Autodesk Inventor part; units mm, degrees
ref_plane "YZ Plane" through (0, 0, 0) normal (1, 0, 0) x (0, 1, 0)
ref_plane "XZ Plane" through (0, 0, 0) normal (0, 1, 0) x (-1, 0, 0)
ref_plane "XY Plane" through (0, 0, 0) normal (0, 0, 1) x (1, 0, 0)
sketch "Sketch1" plane through (0, 0, 0) normal (0, 0, 1) x (1, 0, 0)
  line L0 (-17.5, 16) -> (17.5, 16)
  line L1 (17.5, 16) -> (17.5, -16)
  line L2 (17.5, -16) -> (-17.5, -16)
  line L3 (-17.5, -16) -> (-17.5, 16)
  point P0 (0, 0)
  dimension "d0" = 35
  dimension "d1" = 32
  dimension "d2" = 16
  dimension "d3" = 17.5
extrude "Extrusion1" add sketch "Sketch1" along normal blind 30
sketch "Sketch2" plane through (-17.5, 16, 0) normal (0, 1, 0) x (1, 0, 0)
  line L0 (0, 0) -> (35, 0)
  line L1 (0, 0) -> (0, -30)
  line L2 (35, -30) -> (0, -30)
  line L3 (35, 0) -> (35, -30)
  line L4 (0, 0) -> (0, -30)
  line L5 (35, 0) -> (35, -30)
  line L6 (0, 0) -> (35, 0)
  line L7 (35, 0) -> (35, -8)
  line L8 (35, -8) -> (0, -8)
  line L9 (0, -8) -> (0, 0)
  point P0 (17.5, 0)
  dimension "d6" = 8
extrude "Extrusion2" add sketch "Sketch2" along normal blind 35 contours L0 L3 L8 L1
sketch "Sketch3" plane through (0, 0, 0) normal (0, 0, -1) x (-1, 0, 0)
  circle A0 centre (1.75, -8) radius 0.7835
  circle A1 centre (1.75, 9) radius 0.7835
  point P0 (0, 0)
hole "Hole1" at (-1.75, 9, 0) at (-1.75, -8, 0) direction (0, 0, 1) diameter 2.4 end through all counterbore diameter 4.4 counterbore depth 23
sketch "Sketch4" plane through (17.5, -16, 30) normal (1, 0, 0) x (0, 0, -1)
  line L0 (30, 67) -> (30, 0)
  line L1 (22, 67) -> (30, 67)
  line L2 (22, 32) -> (22, 67)
  line L3 (22, 32) -> (0, 32)
  line L4 (0, 0) -> (0, 32)
  line L5 (30, 0) -> (0, 0)
  point P0 (30, 16)
extrude "Extrusion3" add sketch "Sketch4" along normal blind 15
sketch "Sketch7" plane through (0, 0, 30) normal (0, 0, 1) x (1, 0, 0)
  circle A0 centre (-1.75, 9) radius 1.2
  circle A1 centre (-1.75, -8) radius 1.2
  line L0 (-17.5, 16) -> (32.5, 16)
  line L1 (-17.5, 16) -> (-17.5, -16)
  line L2 (-17.5, -16) -> (32.5, -16)
  line L3 (32.5, 16) -> (32.5, -16)
  line L4 (-6.75, -9) -> (-6.75, -5)
  line L5 (-4.75, -3) -> (1.25, -3)
  line L6 (3.25, -5) -> (3.25, -9)
  line L7 (5.25, -11) -> (25.5, -11)
  line L8 (27.5, -9) -> (27.5, 9)
  line L9 (25.5, 11) -> (5.25, 11)
  line L10 (3.25, 9) -> (3.25, 6)
  line L11 (1.25, 4) -> (-4.75, 4)
  line L12 (-6.75, 6) -> (-6.75, 9)
  line L13 (-8.75, 11) -> (-10.5, 11)
  line L14 (-12.5, 9) -> (-12.5, -9)
  line L15 (-10.5, -11) -> (-8.75, -11)
  arc A2 (-4.75, -3) -> (-6.75, -5) centre (-4.75, -5) ccw
  arc A3 (-8.75, -11) -> (-6.75, -9) centre (-8.75, -9) ccw
  arc A4 (-12.5, -9) -> (-10.5, -11) centre (-10.5, -9) ccw
  arc A5 (-10.5, 11) -> (-12.5, 9) centre (-10.5, 9) ccw
  arc A6 (-6.75, 9) -> (-8.75, 11) centre (-8.75, 9) ccw
  arc A7 (-6.75, 6) -> (-4.75, 4) centre (-4.75, 6) ccw
  arc A8 (1.25, 4) -> (3.25, 6) centre (1.25, 6) ccw
  arc A9 (5.25, 11) -> (3.25, 9) centre (5.25, 9) ccw
  arc A10 (27.5, 9) -> (25.5, 11) centre (25.5, 9) ccw
  arc A11 (25.5, -11) -> (27.5, -9) centre (25.5, -9) ccw
  arc A12 (3.25, -9) -> (5.25, -11) centre (5.25, -9) ccw
  arc A13 (3.25, -5) -> (1.25, -3) centre (1.25, -5) ccw
  point P0 (0, 0)
  point P1 (3.25, 11)
  point P2 (3.25, 4)
  point P3 (-6.75, 4)
  point P4 (-6.75, 11)
  point P5 (-12.5, -11)
  dimension "d18" = 5
  dimension "d19" = 5
  dimension "d21" = 5
  dimension "d22" = 5
  dimension "d23" = 5
  dimension "d24" = 5
  dimension "d25" = 5
  dimension "d26" = 5
  dimension "d27" = 5
  dimension "d28" = 2
  dimension "d29" = 2
extrude "Extrusion4" cut sketch "Sketch7" against normal blind 20 contours A3 L15 A4 L14 A5 L13 A6 L12 A7 L11 A8 L10 A9 L9 A10 L8 A11 L7 A12 L6 A13 L5 A2 L4
properties part number "zgalvo_cover"
Work out the finished part from the listing and answer in its coordinate system (mm). A direction names the side the tool comes from. Round coordinates to 2 decimals unless told otherwise and drop trailing zeros. Write each loop counter-clockwise with the first axis right and the second up, starting at its lowest first coordinate (ties: lowest second). Pieces come first, ordered by that corner, then holes. Notation, with made-up numbers: M 30.5,78.25 L 70.5,78.25 A24 ccw 70.5,110.25 Z; hole C 65,-40 d10. An arc over 180 degrees is marked long. Use a Markdown table: item, result.
1) The part is cut by section A-A on z = 25.25. State how many separate pieces and enclosed holes the cut face has, plus the area to 3 significant figures.
Taken from the geometry:
| item | result |
|---|---|
| separate pieces | 1 |
| enclosed holes | 3 |
| area | 864 mm2 |
2) Which of the six approach directions +Z, -Z, +X, -X, +Y, -Y give full straight-line access (tool end or side, diameter ignored) to faces 4 (the face through (0, -8, 23)), 5 (the face through (3.82, -10.4, 20.14)), 6 (the face through (32.5, 3, 12))?
Taken from the geometry:
| item | result |
|---|---|
| face 4 | -Z |
| face 5 | +Z |
| face 6 | +Z, -Z, +X, +Y, -Y |
3) The part is cut by section B-B on x = -1.75. Give the vertices of the cut face in (y, z).
Taken from the geometry:
| item | result |
|---|---|
| outline | M -16,0 L -10.2,0 L -10.2,23 L -9.2,23 L -9.2,30 L -16,30 Z; M -6.8,23 L -5.8,23 L -5.8,0 L 6.8,0 L 6.8,23 L 7.8,23 L 7.8,30 L 4,30 L 4,10 L -3,10 L -3,30 L -6.8,30 Z; M 10.2,23 L 11.2,23 L 11.2,0 L 51,0 L 51,8 L 16,8 L 16,30 L 10.2,30 Z |
4) Determine the mould class of faces 1 (the face through (7, 51, 4)), 2 (the face through (7, 18, 0)), 3 (the face through (3.85, 10.43, 20.14)) for opening direction Y: pulls with the +Y half, pulls with the -Y half, needs draft (parallel to the pull), parting line crosses it, or undercut.
Taken from the geometry:
| item | result |
|---|---|
| face 1 | pulls with the +Y half |
| face 2 | needs draft |
| face 3 | undercut |
5) Flat-ended cylindrical pins translate along their axes: pin 1 (12 mm diameter, centred on x = 2.5, z = 18, fed in from +Y); pin 2 (11 mm diameter, centred on x = 17.5, y = -2.5, fed in from +Z); pin 3 (1 mm diameter, centred on x = -2.5, y = 28, fed in from +Z). Find the tip coordinate at first contact, or state that the pin passes through.
Taken from the geometry:
| item | result |
|---|---|
| pin 1 | stops at y = 16 |
| pin 2 | stops at z = 10 |
| pin 3 | stops at z = 8 |
6) The part is cut by section C-C on y = -8. Give the vertices of the cut face in (x, z).
Taken from the geometry:
| item | result |
|---|---|
| outline | M -17.5,0 L -3.95,0 L -3.95,23 L -2.95,23 L -2.95,30 L -6.75,30 L -6.75,10 L -12.5,10 L -12.5,30 L -17.5,30 Z; M -0.55,23 L 0.45,23 L 0.45,0 L 32.5,0 L 32.5,30 L 27.5,30 L 27.5,10 L 3.25,10 L 3.25,30 L -0.55,30 Z |
7) Consider line 1 (Y direction, x = -1.75, z = 28.75); line 2 (X direction, y = 9, z = 28.75); line 3 (Y direction, x = -1.75, z = 14.5). Determine where each line is inside the solid, lowest interval first. Write a range as [from, to].
Taken from the geometry:
| item | result |
|---|---|
| line 1 | y = [-16, -9.2], [-6.8, -3], [4, 7.8], [10.2, 16] |
| line 2 | x = [-17.5, -12.5], [-6.75, -2.95], [-0.55, 3.25], [27.5, 32.5] |
| line 3 | y = [-16, -10.2], [-5.8, -3], [4, 6.8], [11.2, 16] |
